The model under review builds one solid part; all positions refer to its coordinate system, in mm. A direction names the side the tool comes from. Give positions to 0.01 mm unless a question says otherwise; leave off trailing zeros. Loops run counter-clockwise (first coordinate to the right, second up) from the corner with the lowest first, then second, coordinate; pieces in that order, holes last. Notation, with made-up numbers: (12, 81) - (18, 81) arc R32 ccw to (18, 107) - close; hole circle Ø5 at (48.5, 68.5). An arc over 180 degrees is marked (long way). Return JSON: item names as keys, results as strings. Group by question number.
from build123d import *

# Parameters (mm, degrees)
CUT_EXTRUDE1_DEPTH      = 125.655525349
CUT_EXTRUDE1_DEPTH_BACK = 125.655525349
SKETCH2_R               = 8


with BuildPart() as part:
    # Sketch1 → Revolve1 (revolve)
    with BuildSketch(Plane.XY, mode=Mode.PRIVATE) as revolve1_sk:
        with BuildLine():
            Line((38, 23.139710977), (38, 0))
            Line((38, 0), (48, 0))
            Line((48, 0), (48, 35.560066311))
            ThreePointArc((48, 35.560066311), (45.832590181, 40.792656492), (40.6, 42.960066311))
            Line((40.6, 42.960066311), (40.4, 42.960066311))
            ThreePointArc((40.4, 42.960066311), (35.167409819, 45.127476131), (33, 50.360066311))
            Line((33, 50.360066311), (33, 83))
            ThreePointArc((33, 83), (32.414213562, 84.414213562), (31, 85))
            Line((31, 85), (23, 85))
            Line((23, 85), (23, 45))
            Line((23, 45), (0, 45))
            Line((0, 45), (0, 39))
            Line((0, 39), (32.515260934, 30.287562091))
            ThreePointArc((32.515260934, 30.287562091), (36.470814718, 27.644545551), (38, 23.139710977))
        make_face()
    revolve(revolve1_sk.sketch.rotate(Axis((0, 0, 0), (1, 0, 0)), 90), axis=Axis((0, 0, 0), (1, 0, 0)))

    # Sketch2 → Cut-Extrude1 (cut, two sides: drawn at the far end of the back side and taken through both)
    with BuildSketch(Plane(origin=(33, 0, 0), x_dir=(0, 0, -1), z_dir=(1, 0, 0)).offset(-CUT_EXTRUDE1_DEPTH_BACK)):
        with Locations((70, 0)):
            Circle(SKETCH2_R)
        with Locations((35, -60.621778265)):
            Circle(SKETCH2_R)
        with Locations((-35, -60.621778265)):
            Circle(SKETCH2_R)
        with Locations((-70, 0)):
            Circle(SKETCH2_R)
        with Locations((-35, 60.621778265)):
            Circle(SKETCH2_R)
        with Locations((35, 60.621778265)):
            Circle(SKETCH2_R)
    extrude(amount=CUT_EXTRUDE1_DEPTH + CUT_EXTRUDE1_DEPTH_BACK, mode=Mode.SUBTRACT)


solid = part.part
Item 1: Tool access review of faces 4 (the face through (0, -37, -14)), 5 (the face through (33, 36, -36)), 6 (the face through (38, 0, 0)): name each direction out of +Z, -Z, +X, -X, +Y, -Y from which nothing blocks a thin tool from reaching the whole face with its end or side.
Item 2: For L1, parallel to Y at x = 27.5, z = 35; L2, parallel to Z at x = 32, y = -1; L3, parallel to Z at x = 21, y = -8, list the stretches that pass through material, from the lowest coordinate up. Write a range as from..to.
Item 3: Mouldability with a two-part tool opening along Y and no side actions: class faces 1 (the face through (27.93, -4.868, 76.349)), 2 (the face through (23, 37, 37)), 3 (the face through (26.944, -25.532, 81.075)) as +Y half, -Y half, draft (parallel to the pull), parting line (faces both ways), or undercut.
Item 4: For P1, Ø21, axis at y = 0, z = 70, coming from the -X side; P2, Ø6, axis at x = 33, y = 40, coming from the -Z side; P3, Ø14, axis at y = -11.5, z = 11.5, coming from the -X side, all flat-tipped, find the tip position at first contact; note any pin that passes through.
Item 5: Take a section at C-C (x = 11). State the section outline as (y, z) points.
Item 6: Take a section at A-A (y = 0). State how many separate pieces and enclosed holes the cut face has, then the cut area to 3 significant figures.
Item 7: Take a section at B-B (z = 0). State the section outline as (x, y) points, then the cut area to 3 significant figures.
Check sheet entries:
{
 "1": {"face 4": "+Z, -Z, -X, +Y, -Y", "face 5": "+X", "face 6": "-X"},
 "2": {"L1": "y = -77.46..-68.62, -52.62..52.62, 68.62..77.46", "L2": "z = -84.73..-77.94, -62.06..-30.41, 30.41..62.06, 77.94..84.73", "L3": "z = -44.28..-32.4, 32.4..44.28"},
 "3": {"face 1": "undercut", "face 2": "draft", "face 3": "parting line"},
 "4": {"P1": "stops at x = 23", "P2": "stops at z = -76.26", "P3": "stops at x = 38"},
 "5": {"outline": "circle Ø90 at (0, 0); hole circle Ø72.11 at (0, 0)"},
 "6": {"separate pieces": "3", "enclosed holes": "0", "area": "2,170 mm^2"},
 "7": {"outline": "(0, -45) - (23, -45) - (23, -85) - (31, -85) arc R2 ccw to (33, -83) - (33, -50.36) arc R7.4 cw to (40.4, -42.96) - (40.6, -42.96) arc R7.4 ccw to (48, -35.56) - (48, 35.56) arc R7.4 ccw to (40.6, 42.96) - (40.4, 42.96) arc R7.4 cw to (33, 50.36) - (33, 83) arc R2 ccw to (31, 85) - (23, 85) - (23, 45) - (0, 45) - (0, 39) - (32.52, 30.29) arc R7.4 cw to (38, 23.14) - (38, -23.14) arc R7.4 cw to (32.52, -30.29) - (0, -39) - close", "area": "2,490 mm^2"}
}
